```python
from build123d import *

# Parameters (mm, degrees)
SKETCH_1_W          = 102
SKETCH_1_H          = 49
EXTRUDE_1_DEPTH     = 3
SKETCH_2_R          = 1.5
CUT_EXTRUDE_1_DEPTH = 4
SKETCH_3_W          = 62
SKETCH_3_H          = 3
EXTRUDE_2_DEPTH     = 7
FILLET_1_R          = 2
FILLET_2_R          = 2
MM_PRESS_1_D        = 3
SKETCH_6_R          = 3.5
SKETCH_6_W          = 5.5
SKETCH_6_H          = 20
SKETCH_6_W_2        = 7.049620939
SKETCH_6_H_2        = 7.099016596
SKETCH_6_W_3        = 14.194500079
SKETCH_6_H_3        = 6.456669412
CUT_EXTRUDE_2_DEPTH = 7


with BuildPart() as part:
    # 草图1 → 凸台-拉伸1 (new body)
    with BuildSketch(Plane.XY):
        with Locations((82, -24.5)):
            Rectangle(SKETCH_1_W, SKETCH_1_H)
    extrude(amount=EXTRUDE_1_DEPTH)

    # 草图2 → 切除-拉伸1 (cut, through all)
    with BuildSketch(Plane(origin=(0, 0, 0), x_dir=(-1, 0, 0), z_dir=(0, 0, -1))):
        with Locations((-130, -46)):
            Circle(SKETCH_2_R)
        with Locations((-130, -3)):
            Circle(SKETCH_2_R)
        with Locations((-34, -3)):
            Circle(SKETCH_2_R)
        with Locations((-34.5, -15.5)):
            Circle(SKETCH_2_R)
        with Locations((-34, -46)):
            Circle(SKETCH_2_R)
        with Locations((-34.5, -33.5)):
            Circle(SKETCH_2_R)
    extrude(amount=-CUT_EXTRUDE_1_DEPTH, mode=Mode.SUBTRACT)

    # 草图3 → 凸台-拉伸2 (add)
    with BuildSketch(Plane(origin=(0, 0, 0), x_dir=(-1, 0, 0), z_dir=(0, 0, -1))):
        with Locations((-80, -11.6)):
            Rectangle(SKETCH_3_W, SKETCH_3_H)
        with Locations((-80, -37.4)):
            Rectangle(SKETCH_3_W, SKETCH_3_H)
    extrude(amount=EXTRUDE_2_DEPTH)

    # 圆角1
    fillet_1_edges = [part.edges().sort_by_distance(p)[0] for p in [
        (80, -13.1, 0),
    ]]
    fillet(fillet_1_edges, radius=FILLET_1_R)

    # 圆角2
    fillet_2_edges = [part.edges().sort_by_distance(p)[0] for p in [
        (80, -35.9, 0),
    ]]
    fillet(fillet_2_edges, radius=FILLET_2_R)

    # 大小mm Press 暗销孔1 (through all)
    with Locations(Plane(origin=(43.000752307, -10.1, 120.302802184), x_dir=(0.99978014, 0, -0.020968354), z_dir=(0, 1, 0))):
        with Locations((20.591231353, 123.39816829), (42.591231353, 122.936763059), (64.581557509, 122.475560716)):
            Hole(MM_PRESS_1_D / 2)

    # 草图6 → 切除-拉伸2 (cut)
    with BuildSketch(Plane.XY.offset(3)):
        with Locations((127, -14)):
            Circle(SKETCH_6_R)
        with Locations((127, -35)):
            Circle(SKETCH_6_R)
        with Locations((108.159552583, -24.5)):
            Rectangle(SKETCH_6_W, SKETCH_6_H)
        with Locations((46.525562777, -24.5)):
            Rectangle(SKETCH_6_W_2, SKETCH_6_H_2)
        with Locations((120.733739183, -24.5)):
            Rectangle(SKETCH_6_W_3, SKETCH_6_H_3)
    extrude(amount=-CUT_EXTRUDE_2_DEPTH, mode=Mode.SUBTRACT)


solid = part.part
```
The listing builds one solid part. Answer for the finished solid, in the listing's coordinates (mm). A direction names the side the tool comes from. Round coordinates to 2 decimals unless told otherwise and drop trailing zeros. Loops run counter-clockwise (first coordinate to the right, second up) from the corner with the lowest first, then second, coordinate; pieces in that order, holes last.
Q1. Find the intervals of material crossed by line 1 (Y direction, x = 127, z = 0.7); line 2 (X direction, y = -37.5, z = -3.5); line 3 (Y direction, x = 89.5, z = -3), in increasing order.
Q2. Section D-D, the plane z = 1 is taken. Count the separate pieces of the cut face and the enclosed holes in it, then the cut area to 3 significant figures.
Q3. Section B-B, the plane x = 48 is taken. Determine the outline of the cut face in (y, z).
Q4. Section A-A, the plane y = -3 is taken. Determine the outline of the cut face in (x, z).
Q5. Which of the six approach directions +Z, -Z, +X, -X, +Y, -Y give full straight-line access (tool end or side, diameter ignored) to faces 5 (the face through (80, -10.1, -3)), 6 (the face through (121, -27.728, 2)), 7 (the face through (103.56, -37.42, -3.92)), 8 (the face through (80, -13.1, -4)), 9 (the face through (49, -38, -3))?
Q6. Given pin 1 Ø9 at (x, y) = (127, -35) entering from -Z; pin 2 Ø1 at (x, z) = (54, -1) entering from -Y; pin 3 Ø2.5 at (y, z) = (-35.5, -4.5) entering from +X, each flat-ended and moving along its own axis, determine where each tip first touches the part or whether it passes through.
Q7. For a pull along X with two mould halves and no side action, classify faces 1 (the face through (108, -14.5, 1)), 2 (the face through (46, -28.05, 2)), 3 (the face through (80, -38.9, -3)), 4 (the face through (111, -12, -3)) as released by +X, released by -X, zero draft, split by the parting line, or undercut.
Q8. Section C-C, the plane x = 34 is taken. Determine the outline of the cut face in (y, z).
Completed:
1. line 1: y = -49 to -38.5, -31.5 to -27.73, -21.27 to -17.5, -10.5 to 0
1. line 2: x = 49 to 59.5, 62.5 to 81.5, 84.5 to 103.5, 106.5 to 111
1. line 3: y = -38.9 to -35.9, -13.1 to -10.1
2. separate pieces: 1
2. enclosed holes: 11
2. area: 4,630 mm2
3. outline: (-49, 0) - (-28.05, 0) - (-28.05, 3) - (-49, 3) - close; (-20.95, 0) - (0, 0) - (0, 3) - (-20.95, 3) - close
4. outline: (31, 0) - (32.5, 0) - (32.5, 3) - (31, 3) - close; (35.5, 0) - (128.5, 0) - (128.5, 3) - (35.5, 3) - close; (131.5, 0) - (133, 0) - (133, 3) - (131.5, 3) - close
5. face 5: -Z, +X, -X, +Y
5. face 6: +Z, -Z
5. face 7: +Y, -Y
5. face 8: -Z, +X, -X
5. face 9: -Z, -X, +Y, -Y
6. pin 1: stops at z = 0
6. pin 2: stops at y = -38.9
6. pin 3: stops at x = 111
7. face 1: undercut
7. face 2: undercut
7. face 3: zero draft
7. face 4: released by +X
8. outline: (-49, 0) - (-47.5, 0) - (-47.5, 3) - (-49, 3) - close; (-44.5, 0) - (-34.91, 0) - (-34.91, 3) - (-44.5, 3) - close; (-32.09, 0) - (-16.91, 0) - (-16.91, 3) - (-32.09, 3) - close; (-14.09, 0) - (-4.5, 0) - (-4.5, 3) - (-14.09, 3) - close; (-1.5, 0) - (0, 0) - (0, 3) - (-1.5, 3) - close
